Here's how the part is built. I have some questions about the finished solid (model axes, mm). Face numbers are marked on the shaded views. Round coordinates to 2 decimals unless told otherwise and drop trailing zeros. Write each loop counter-clockwise with the first axis right and the second up, starting at its lowest first coordinate (ties: lowest second). Pieces come first, ordered by that corner, then holes. Notation, with made-up numbers: (2.5, 76) -> (10.5, 76) arc R27 cw to (10.5, 106) -> close; hole circle Ø6 at (-8.75, -5). An arc over 180 degrees is marked (long way). Answer in a Markdown table with one row per item.
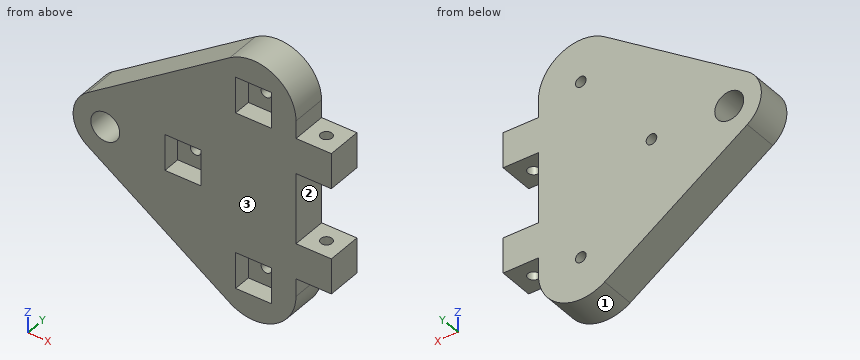
from build123d import *

# Parameters (mm, degrees)
SKETCH_1_R               = 4.1
EXTRUDE_1_DEPTH          = 10
SKETCH_2_W               = 10.2
SKETCH_2_H               = 10.2
CUT_EXTRUDE_1_DEPTH      = 5
SKETCH_3_W               = 10
SKETCH_3_H               = 10
EXTRUDE_2_DEPTH          = 10
CUT_EXTRUDE_2_DEPTH      = 64.876521508
CUT_EXTRUDE_2_DEPTH_BACK = 64.876521508
SKETCH_4_R               = 1.6
SKETCH_5_R               = 1.5
CUT_EXTRUDE_3_DEPTH      = 64.876521508


with BuildPart() as part:
    # ｽｹｯﾁ1 → ﾎﾞｽ - 押し出し1 (new body)
    with BuildSketch(Plane(origin=(0, 0, 0), x_dir=(1, 0, 0), z_dir=(0, 1, 0))):
        with BuildLine():
            Line((-47.110254718, 7.529627927), (-6.738797431, 34.929179684))
            ThreePointArc((-6.738797431, 34.929179684), (5.618470914, 35.603432679), (12, 25))
            Line((12, 25), (12, -25))
            ThreePointArc((12, -25), (5.618470914, -35.603432679), (-6.738797431, -34.929179684))
            Line((-6.738797431, -34.929179684), (-47.110254718, -7.529627927))
            ThreePointArc((-47.110254718, -7.529627927), (-51.1, 0), (-47.110254718, 7.529627927))
        make_face()
        with Locations(Location((-42, 0, 0), (0, 0, 270))):
            Circle(SKETCH_1_R, mode=Mode.SUBTRACT)
    extrude(amount=EXTRUDE_1_DEPTH)

    # ｽｹｯﾁ2 → ｶｯﾄ - 押し出し1 (cut)
    with BuildSketch(Plane.XZ):
        with Locations((0, 25)):
            Rectangle(SKETCH_2_W, SKETCH_2_H)
        with Locations((0, -25)):
            Rectangle(SKETCH_2_W, SKETCH_2_H)
        with Locations((-20, 0)):
            Rectangle(SKETCH_2_W, SKETCH_2_H)
    extrude(amount=-CUT_EXTRUDE_1_DEPTH, mode=Mode.SUBTRACT)

    # ｽｹｯﾁ3 → ﾎﾞｽ - 押し出し2 (add)
    with BuildSketch(Plane(origin=(12, 0, 0), x_dir=(0, 0, -1), z_dir=(1, 0, 0))):
        with Locations((-15, 5)):
            Rectangle(SKETCH_3_W, SKETCH_3_H)
        with Locations((15, 5)):
            Rectangle(SKETCH_3_W, SKETCH_3_H)
    extrude(amount=EXTRUDE_2_DEPTH)

    # ｽｹｯﾁ4 → ｶｯﾄ - 押し出し2 (cut, two sides: drawn at the far end of the back side and taken through both)
    with BuildSketch(Plane.XY.offset(-CUT_EXTRUDE_2_DEPTH_BACK)):
        with Locations((17, 5)):
            Circle(SKETCH_4_R)
    extrude(amount=CUT_EXTRUDE_2_DEPTH + CUT_EXTRUDE_2_DEPTH_BACK, mode=Mode.SUBTRACT)

    # ｽｹｯﾁ5 → ｶｯﾄ - 押し出し3 (cut, through all)
    with BuildSketch(Plane(origin=(0, 0, 0), x_dir=(1, 0, 0), z_dir=(0, 1, 0))):
        with Locations(Location((0, -25, 0), (0, 0, 270))):
            Circle(SKETCH_5_R)
        with Locations(Location((-20, 0, 0), (0, 0, 270))):
            Circle(SKETCH_5_R)
        with Locations(Location((0, 25, 0), (0, 0, 90))):
            Circle(SKETCH_5_R)
    extrude(amount=CUT_EXTRUDE_3_DEPTH, mode=Mode.SUBTRACT)


solid = part.part
1) I want a section at C-C, the plane x = 17. List the corners of the cut face in (y, z) for me, and give its area (3 significant figures).
Response:
| item | result |
|---|---|
| outline | (0, -20) -> (3.4, -20) -> (3.4, -10) -> (0, -10) -> close; (0, 10) -> (3.4, 10) -> (3.4, 20) -> (0, 20) -> close; (6.6, -20) -> (10, -20) -> (10, -10) -> (6.6, -10) -> close; (6.6, 10) -> (10, 10) -> (10, 20) -> (6.6, 20) -> close |
| area | 136 mm^2 |
2) We'd pull the mould along Z, two halves only. Please class the marked faces 1, 2 and 3: +Z half, -Z half, draft (parallel to the pull), parting line (faces both ways), or undercut.
Response:
| item | result |
|---|---|
| face 1 | -Z half |
| face 2 | undercut |
| face 3 | draft |
3) For pin 1 (1.5 mm diameter, centred on y = 3.5, z = -21.5, fed in from +X); pin 2 (2.5 mm diameter, centred on x = -2.5, y = 2.5, fed in from +Z); pin 3 (2 mm diameter, centred on x = -40.5, y = 5.5, fed in from -Z), each with a flat end and sliding along its axis, tell me the tip position at first contact or that it passes through.
Response:
| item | result |
|---|---|
| pin 1 | stops at x = 12 |
| pin 2 | stops at z = 36.93 |
| pin 3 | stops at z = -12.69 |
4) I want a section at D-D, the plane z = -18. List the corners of the cut face in (x, y) for me, and give its area (3 significant figures).
Response:
| item | result |
|---|---|
| outline | (-31.68, 0) -> (22, 0) -> (22, 10) -> (-31.68, 10) -> close; hole circle Ø3.2 at (17, 5) |
| area | 529 mm^2 |
5) I want a section at B-B, the plane y = 1. List the corners of the cut face in (x, z) for me, and give its area (3 significant figures).
Response:
| item | result |
|---|---|
| outline | (-47.11, -7.53) -> (-6.74, -34.93) arc R12 ccw to (12, -25) -> (12, -20) -> (22, -20) -> (22, -10) -> (12, -10) -> (12, 10) -> (22, 10) -> (22, 20) -> (12, 20) -> (12, 25) arc R12 ccw to (-6.74, 34.93) -> (-47.11, 7.53) arc R9.1 ccw to start; hole circle Ø8.2 at (-42, 0); hole (-25.1, -5.1) -> (-14.9, -5.1) -> (-14.9, 5.1) -> (-25.1, 5.1) -> close; hole (-5.1, -30.1) -> (5.1, -30.1) -> (5.1, -19.9) -> (-5.1, -19.9) -> close; hole (-5.1, 19.9) -> (5.1, 19.9) -> (5.1, 30.1) -> (-5.1, 30.1) -> close |
| area | 2,910 mm^2 |
6) I need wall thicknesses on line 1 (X direction, y = 7.5, z = 0); line 2 (Z direction, x = 0.5, y = 1.25); line 3 (X direction, y = 4.25, z = 0). Which ranges of each line are inside material? Lowest first, please. Write a range as [from, to].
Response:
| item | result |
|---|---|
| line 1 | x = [-51.1, -46.1], [-37.9, -21.5], [-18.5, 12] |
| line 2 | z = [-36.99, -30.1], [-19.9, 19.9], [30.1, 36.99] |
| line 3 | x = [-51.1, -46.1], [-37.9, -25.1], [-14.9, 12] |
7) I want a section at A-A, the plane x = 0. List the corners of the cut face in (y, z) for me.
Response:
| item | result |
|---|---|
| outline | (0, -37) -> (10, -37) -> (10, -26.5) -> (5, -26.5) -> (5, -30.1) -> (0, -30.1) -> close; (0, -19.9) -> (5, -19.9) -> (5, -23.5) -> (10, -23.5) -> (10, 23.5) -> (5, 23.5) -> (5, 19.9) -> (0, 19.9) -> close; (0, 30.1) -> (5, 30.1) -> (5, 26.5) -> (10, 26.5) -> (10, 37) -> (0, 37) -> close |
